Autodesk Inventor part; units mm, degrees
ref_plane "YZ Plane" through (0, 0, 0) normal (1, 0, 0) x (0, 1, 0)
ref_plane "XZ Plane" through (0, 0, 0) normal (0, 1, 0) x (-1, 0, 0)
ref_plane "XY Plane" through (0, 0, 0) normal (0, 0, 1) x (1, 0, 0)
sketch "Sketch1" plane through (0, 0, 0) normal (0, 0, 1) x (1, 0, 0)
  line L0 (0, 0) -> (49.8, 0)
  line L1 (49.8, 0) -> (49.8, 30.921)
  line L2 (49.8, 30.921) -> (0, 30.921)
  line L3 (0, 30.921) -> (0, 0)
  dimension "d0" = 49.8
  dimension "d1" = 30.921
extrude "Extrusion1" add sketch "Sketch1" along normal blind 5
sketch "Sketch3" plane through (0, 0, 5) normal (0, 0, 1) x (1, 0, 0)
  line L0 (0, 0) -> (49.8, 0)
  line L1 (24.9, 0) -> (41.821, 0) construction
  line L2 (49.8, 0) -> (49.8, 30.921)
  line L3 (22.9, 16.921) -> (26.9, 16.921)
  line L4 (24.9, 14.921) -> (24.9, 18.921)
  circle A0 centre (24.9, 16.921) radius 2
  dimension "d22" = 4
  dimension "d23" = 4
  dimension "d24" = 4
  dimension "d25" = 16.921
  dimension "d26" = 24.9
sketch "Sketch4" plane through (0, 0, 5) normal (0, 0, 1) x (1, 0, 0)
  line L0 (0, 0) -> (49.8, 0)
  line L1 (0, 0) -> (7.1085, 7.1085)
  line L2 (0, 0) -> (10.053, 0) construction
  line L3 (17.8214, 5.3223) -> (45.7841, 5.3223) construction
  line L4 (22.1418, 11.0415) -> (25.8541, 14.7538)
  line L5 (25.8541, 14.7538) -> (23.7328, 16.8751)
  line L6 (23.7328, 16.8751) -> (20.0205, 13.1628)
  line L7 (20.0205, 13.1628) -> (22.1418, 11.0415)
  line L8 (16.6871, 14.6491) -> (21.9371, 14.6491) construction
  line L9 (20.0205, 13.1628) -> (25.8541, 14.7538)
  line L10 (23.7328, 16.8751) -> (22.1418, 11.0415)
  line L11 (22.9373, 13.9583) -> (23.9979, 12.8976)
  line L12 (22.9, 16.921) -> (26.9, 16.921)
  line L13 (24.9, 14.921) -> (24.9, 18.921)
  circle A0 centre (24.9, 16.921) radius 2
  line L14 (22.8984, 10.2849) -> (26.6107, 13.9972)
  line L15 (6.9567, 4.2426) -> (27.8163, 25.1023)
  line L16 (32.6954, 20.2233) -> (64.1581, 20.2233) construction
  circle A1 centre (30.6448, 19.799) radius 0.75
  circle A2 centre (10.4922, 2.4749) radius 0.75
  line L17 (31.2069, 17.1792) -> (24.8429, 23.5431)
  line L18 (12.9989, 11.6991) -> (19.3629, 5.3351)
  line L19 (26.6107, 13.9972) -> (32.7661, 20.1525)
  line L20 (20.6107, 13.9972) -> (29.3157, 13.9972) construction
  line L21 (32.7661, 20.1525) -> (11.9064, -0.7071)
  line L22 (11.9064, -0.7071) -> (6.9567, 4.2426)
  line L23 (27.8163, 25.1023) -> (32.7661, 20.1525)
  line L24 (29.0217, 22.4081) -> (58.5217, 22.4081) construction
  line L25 (12.9989, 11.6991) -> (24.8429, 23.5431)
  line L26 (31.2069, 17.1792) -> (19.3629, 5.3351)
  line L27 (14.162, 1.5485) -> (11.9064, -0.7071)
  line L28 (10.9064, -0.7071) -> (14.0963, -0.7071) construction
  line L29 (10.8458, 2.8284) -> (10.4922, 2.4749)
  line L30 (10.8458, 2.8284) -> (11.3458, 2.8284) construction
  line L31 (10.9064, -0.7071) -> (11.9064, -0.7071)
  circle A3 centre (30.6448, 19.799) radius 0.6
  circle A4 centre (10.4922, 2.4749) radius 0.6
  point P0 (25.55, 22.836)
  point P1 (13.706, 10.992)
  dimension "d27" = 10.053
  dimension "d28" = 45
  dimension "d32" = 5.25
  dimension "d33" = 45
  dimension "d34" = 3
  dimension "d36" = 1.07
  dimension "d40" = 1.5
  dimension "d43" = 1.5
  dimension "d46" = 5.5
  dimension "d47" = 6
  dimension "d51" = 8.705
  dimension "d52" = 45
  dimension "d53" = 29.5
  dimension "d54" = 135
  dimension "d55" = 7
  dimension "d56" = 3.75
  dimension "d57" = 1
  dimension "d58" = 1
  dimension "d59" = 2.93
  dimension "d60" = 1.25
  dimension "d61" = 1.75
  dimension "d97" = 135
  dimension "d98" = 0.5
  dimension "d99" = 135
  dimension "d101" = 1
  dimension "d102" = 1.2
  dimension "d103" = 1.2
extrude "Extrusion3" cut sketch "Sketch4" against normal blind 5 contours L18 L25 L17 L15 | L15 L17 L19 L14 L21 L18 | L21 L14 L19 L17 L26 L18 | L10 L11 L4 | L7 L9 L10 | L11 L9 L4 | L6 A0 L10 L9 | L10 A0 L5 L9 | A0 L12 L13 L5 L6 | L6 L10 A0 | L10 L5 L13 A0 | A0 L13 L5 | L5 L13 L12 A0 | A0 L13 L12 | L12 L13 A0 | A3 | A4
sketch "Sketch5" plane through (0, 0, 5) normal (0, 0, 1) x (1, 0, 0)
  circle A0 centre (4.9, 26.921) radius 1.55
  circle A1 centre (44.9, 7) radius 1.55
  circle A2 centre (44.9, 26.921) radius 1.55
  line L0 (0, 30.921) -> (0, 0)
  line L1 (49.8, 30.921) -> (0, 30.921)
  line L2 (49.8, 0) -> (49.8, 30.921)
  line L3 (0, 0) -> (49.8, 0)
  dimension "d62" = 3.1
  dimension "d63" = 3.1
  dimension "d64" = 3.1
  dimension "d65" = 4.9
  dimension "d66" = 4
  dimension "d67" = 4.9
  dimension "d68" = 4
  dimension "d69" = 4.9
  dimension "d70" = 7
extrude "Extrusion4" cut sketch "Sketch5" against normal blind 5 contours A0 | A1 | A2
sketch "Sketch6" plane through (0, 0, 5) normal (0, 0, 1) x (1, 0, 0)
  circle A0 centre (4.9, 26.921) radius 1.55
  line L0 (2.15, 29.671) -> (7.65, 24.171) construction
  line L1 (7.65, 29.671) -> (2.15, 24.171) construction
  line L2 (3.3975, 24.3186) -> (1.895, 26.921)
  line L3 (1.895, 26.921) -> (3.3975, 29.5234)
  line L4 (3.3975, 29.5234) -> (6.4025, 29.5234)
  line L5 (6.4025, 29.5234) -> (7.905, 26.921)
  line L6 (7.905, 26.921) -> (6.4025, 24.3186)
  line L7 (6.4025, 24.3186) -> (3.3975, 24.3186)
  line L8 (43.3975, 29.5234) -> (46.4025, 29.5234)
  line L9 (41.895, 26.921) -> (43.3975, 29.5234)
  line L10 (43.3975, 24.3186) -> (41.895, 26.921)
  line L11 (46.4025, 24.3186) -> (43.3975, 24.3186)
  line L12 (47.905, 26.921) -> (46.4025, 24.3186)
  line L13 (46.4025, 29.5234) -> (47.905, 26.921)
  line L14 (44.9, 26.921) -> (44.9, 16.921)
  line L15 (43.3975, 4.3976) -> (41.895, 7)
  line L16 (41.895, 7) -> (43.3975, 9.6024)
  line L17 (43.3975, 9.6024) -> (46.4025, 9.6024)
  line L18 (46.4025, 9.6024) -> (47.905, 7)
  line L19 (47.905, 7) -> (46.4025, 4.3976)
  line L20 (46.4025, 4.3976) -> (43.3975, 4.3976)
  point P0 (0, 0)
  point P1 (44.9, 7)
  dimension "d73" = 5.5
  dimension "d74" = 5.5
  dimension "d81" = 6.01
  dimension "d84" = 40
  dimension "d89" = 10
  dimension "d92" = 19.921
extrude "Extrusion5" cut sketch "Sketch6" against normal blind 1.5
properties part number "30_CUBE_penSIM_DMD_Holder"
Design review of the part built by this model. Coordinates are the model's own, in mm. A direction names the side the tool comes from. Give positions to 0.01 mm unless a question says otherwise; leave off trailing zeros. Loops run counter-clockwise (first coordinate to the right, second up) from the corner with the lowest first, then second, coordinate; pieces in that order, holes last. Notation, with made-up numbers: (-25, 7) - (-17, 7) arc R6 cw to (-17, 16) - close; hole circle Ø2 at (-34, 59.25). An arc over 180 degrees is marked (long way). Write item = value, one per line.
1) Take a section at B-B on x = 4.9. State the section outline as (y, z) points, and give its area (3 significant figures).
Result sheet:
outline = (0, 0) - (25.37, 0) - (25.37, 3.5) - (24.32, 3.5) - (24.32, 5) - (0, 5) - close; (28.47, 0) - (30.92, 0) - (30.92, 5) - (29.52, 5) - (29.52, 3.5) - (28.47, 3.5) - close
area = 136 mm2
2) Tool access review of faces 5 (the face through (19, 19, 5)), 6 (the face through (16.1, 8.6, 2.5)), 7 (the face through (47.164, 25.638, 4.26)): name each direction out of +Z, -Z, +X, -X, +Y, -Y from which nothing blocks a thin tool from reaching the whole face with its end or side.
Result sheet:
face_5 = +Z, +X, -X, +Y, -Y
face_6 = +Z, -Z
face_7 = +Z
3) Clearance check with flat-ended pins moving along their axes: pin 1 Ø12 at (x, y) = (25, 12.5) entering from -Z; pin 2 Ø2.5 at (x, y) = (44.9, 7) entering from +Z; pin 3 Ø1.6 at (x, y) = (45.5, 6) entering from +Z. State where each tip first meets the part, or that it passes through.
Result sheet:
pin_1 = 0
pin_2 = through
pin_3 = 3.5
4) Take a section at C-C on y = 11. State the section outline as (x, z) points.
Result sheet:
outline = (0, 0) - (13.7, 0) - (13.7, 5) - (0, 5) - close; (25.03, 0) - (49.8, 0) - (49.8, 5) - (25.03, 5) - close
5) Take a section at A-A on x = 44.9. State the section outline as (y, z) points, and give its area (3 significant figures).
Result sheet:
outline = (0, 0) - (5.45, 0) - (5.45, 3.5) - (4.4, 3.5) - (4.4, 5) - (0, 5) - close; (8.55, 0) - (25.37, 0) - (25.37, 3.5) - (24.32, 3.5) - (24.32, 5) - (9.6, 5) - (9.6, 3.5) - (8.55, 3.5) - close; (28.47, 0) - (30.92, 0) - (30.92, 5) - (29.52, 5) - (29.52, 3.5) - (28.47, 3.5) - close
area = 117 mm2
6) Draft analysis for pull direction X (two halves, no side actions). For faces 1 (the face through (25, 30.921, 2)), 2 (the face through (0, 16, 2)), 3 (the face through (7.143, 28.24, 4.26)), 4 (the face through (7.164, 25.638, 4.26)), state which applies: +X half, -X half, draft (parallel to the pull), parting line (faces both ways), or undercut.
Result sheet:
face_1 = draft
face_2 = -X half
face_3 = undercut
face_4 = undercut
7) Take a section at D-D on z = 4.35. State the section outline as (x, y) points (1 decimal).
Result sheet:
outline = (0, 0) - (49.8, 0) - (49.8, 30.9) - (0, 30.9) - close; hole (1.9, 26.9) - (3.4, 24.3) - (6.4, 24.3) - (7.9, 26.9) - (6.4, 29.5) - (3.4, 29.5) - close; hole circle Ø1.2 at (10.5, 2.5); hole (13, 11.7) - (19.4, 5.3) - (31.2, 17.2) - (24.8, 23.5) - close; hole circle Ø1.2 at (30.6, 19.8); hole (41.9, 7) - (43.4, 4.4) - (46.4, 4.4) - (47.9, 7) - (46.4, 9.6) - (43.4, 9.6) - close; hole (41.9, 26.9) - (43.4, 24.3) - (46.4, 24.3) - (47.9, 26.9) - (46.4, 29.5) - (43.4, 29.5) - close
8) To check wall thickness, follow line 1 (Y direction, x = 44.9, z = 1.05); line 2 (X direction, y = 9, z = 4.5); line 3 (Y direction, x = 4.9, z = 1.6). State the ranges of each line that lie inside material, in increasing order.
Result sheet:
line_1 = 0 to 5.45, 8.55 to 25.37, 28.47 to 30.92
line_2 = 0 to 15.7, 23.03 to 43.05, 46.75 to 49.8
line_3 = 0 to 25.37, 28.47 to 30.92
